Check sheet for the modelled part. Datum: model origin and axes. Units: mm. A direction names the side the tool comes from. Round coordinates to 2 decimals unless told otherwise and drop trailing zeros. Write each loop counter-clockwise with the first axis right and the second up, starting at its lowest first coordinate (ties: lowest second). Pieces come first, ordered by that corner, then holes.
Item 1: Go/stop test with flat-tipped pins: pin 1 Ø1.5 at (y, z) = (5.5, 2.5) entering from +X; pin 2 Ø12.5 at (x, y) = (10.5, -2) entering from -Z; pin 3 Ø2 at (x, z) = (11.5, 2) entering from -Y; pin 4 Ø2.5 at (x, z) = (5.5, 3) entering from +Y. Record where each tip stops, or that it passes through.
Item 2: Cross-section at A-A on x = 0. Enter the section's corners in (y, z), plus the area to 3 significant figures.
Item 3: Cross-section at B-B on z = 8.25. Enter the section's corners in (x, y), plus the area to 3 significant figures.
Item 4: Release check for a two-part mould opening along X. For faces 1 (the flat face through (6, 4.031, 3)), 2 (the cylindrical face through (44.2, -15.6, 6.5)), 3 (the cylindrical face through (20.017, 0.08, 2.958)) record: +X half, -X half, draft (parallel to the pull), parting line (faces both ways), or undercut.
Item 5: Tool access check on faces 4 (the flat face through (43.318, 10.972, 7.521)), 5 (the flat face through (25.915, -11.665, 6.465)), 6 (the cylindrical face through (1.27, -0.97, 7.48)), 7 (the cylindrical face through (0.08, -5.57, 2.96)). Record the directions out of +Z, -Z, +X, -X, +Y, -Y that give a thin tool (end or side, any length) a straight path to the whole face; none if there is none.
Item 6: Cross-section at C-C on y = 0. Enter the section's corners in (x, z).
Item 7: Material ranges on line 1 (Y direction, x = 39.5, z = 7.5); line 2 (Z direction, x = -3.5, y = 1); line 3 (Z direction, x = 17, y = 7), recorded low to high.
from build123d import *

# Parameters (mm, degrees)
BOSS_EXTRUDE1_DEPTH     = 9
BOSS_EXTRUDE2_START     = -5
BOSS_EXTRUDE2_OUTLINE_R = 2.142705637
BOSS_EXTRUDE2_DEPTH     = 5
CUT_EXTRUDE1_DEPTH      = 6
SKETCH9_R               = 1.6
CUT_EXTRUDE2_DEPTH      = 6
CUT_EXTRUDE3_DEPTH      = 3
FILLET1_R               = 1


# Read off the part's stored shape, not the designer's step: Boss-Extrude2
with BuildPart() as part:
    # Sketch2 → Boss-Extrude1 (new body)
    with BuildSketch(Plane.XY):
        with BuildLine():
            Line((13.923486695, -6.250000093), (23.935808117, -6))
            ThreePointArc((23.935808117, -6), (29.935808117, 0), (23.935808117, 6))
            Line((23.935808117, 6), (13.923486695, 6.250000093))
            ThreePointArc((13.923486695, 6.250000093), (9.518581948, 6.542551177), (5.493579732, 8.355871093))
            ThreePointArc((5.493579732, 8.355871093), (-10, 0), (5.493579732, -8.355871093))
            ThreePointArc((5.493579732, -8.355871093), (9.518581948, -6.542551177), (13.923486695, -6.250000093))
        make_face()
    extrude(amount=BOSS_EXTRUDE1_DEPTH)

    # Boss-Extrude2 outline → Boss-Extrude2 (add)
    with BuildSketch(Plane.XY.offset(9).offset(BOSS_EXTRUDE2_START)):
        with BuildLine():
            Line((23.935808117, -6), (13.923486695, -6.250000093))
            Line((13.923486695, -6.250000093), (38.246061815, -17.232807658))
            ThreePointArc((38.246061815, -17.232807658), (44.232088174, -15.557320072), (43.673854661, -9.366347162))
            Line((43.673854661, -9.366347162), (34.3075075, 0))
            Line((34.3075075, 0), (43.673854661, 9.366347162))
            ThreePointArc((43.673854661, 9.366347162), (44.232088174, 15.557320072), (38.246061815, 17.232807658))
            Line((38.246061815, 17.232807658), (13.923486695, 6.250000093))
            Line((13.923486695, 6.250000093), (23.935808117, 6))
            ThreePointArc((23.935808117, 6), (29.935808117, 0), (23.935808117, -6))
        make_face()
        with Locations((40.232073655, -12.797343053)):
            Circle(BOSS_EXTRUDE2_OUTLINE_R, mode=Mode.SUBTRACT)
        with Locations((40.232073655, 12.797343053)):
            Circle(BOSS_EXTRUDE2_OUTLINE_R, mode=Mode.SUBTRACT)
    extrude(amount=BOSS_EXTRUDE2_DEPTH)

    # Sketch7 → Cut-Extrude1 (cut)
    with BuildSketch(Plane(origin=(0, 0, 0), x_dir=(-1, 0, 0), z_dir=(0, 0, -1))):
        with BuildLine():
            ThreePointArc((9.235665873, -3.834380769), (9.999935569, 0.035897224), (9.207899302, 3.900588474))
            Line((9.207899302, 3.900588474), (8.401819085, 4.030860156))
            Line((8.401819085, 4.030860156), (3.901819085, 4.030860156))
            ThreePointArc((3.901819085, 4.030860156), (-0.017364504, 5.630860156), (-3.936548092, 4.030860156))
            Line((-3.936548092, 4.030860156), (-8.436548092, 4.030860156))
            Line((-8.436548092, 4.030860156), (-17.916217693, 2.498838303))
            ThreePointArc((-17.916217693, 2.498838303), (-20.017364504, 0.030860156), (-17.916217693, -2.43711799))
            Line((-17.916217693, -2.43711799), (-8.436548092, -3.969139844))
            Line((-8.436548092, -3.969139844), (-3.936548092, -3.969139844))
            ThreePointArc((-3.936548092, -3.969139844), (-0.017364504, -5.569139844), (3.901819085, -3.969139844))
            Line((3.901819085, -3.969139844), (8.401819085, -3.969139844))
            Line((8.401819085, -3.969139844), (9.235665873, -3.834380769))
        make_face()
    extrude(amount=-CUT_EXTRUDE1_DEPTH, mode=Mode.SUBTRACT)

    # Sketch9 → Cut-Extrude2 (cut)
    with BuildSketch(Plane(origin=(0, 0, 6), x_dir=(-1, 0, 0), z_dir=(0, 0, -1))):
        Circle(SKETCH9_R)
    extrude(amount=-CUT_EXTRUDE2_DEPTH, mode=Mode.SUBTRACT)

    # Sketch10 → Cut-Extrude3 (cut)
    with BuildSketch(Plane.XY.offset(9)):
        Polygon((38.132073655, 9.197343053), (42.332073655, 9.197343053), (44.332073655, 12.797343053), (42.332073655, 16.397343053), (38.132073655, 16.397343053), (36.132073655, 12.797343053), align=None)
        Polygon((38.132073655, -9.197343053), (36.132073655, -12.797343053), (38.132073655, -16.397343053), (42.332073655, -16.397343053), (44.332073655, -12.797343053), (42.332073655, -9.197343053), align=None)
    extrude(amount=-CUT_EXTRUDE3_DEPTH, mode=Mode.SUBTRACT)

    # Fillet1
    fillet1_edges = [part.edges().sort_by_distance(p)[0] for p in [
        (34.3075075, 0, 6.5),
    ]]
    fillet(fillet1_edges, radius=FILLET1_R)


solid = part.part
Response values:
1. pin 1: stops at x = 27.6
1. pin 2: stops at z = 0
1. pin 3: stops at y = -6.34
1. pin 4: stops at y = 9.05
2. outline: (-10, 0) - (-5.57, 0) - (-5.57, 6) - (-1.6, 6) - (-1.6, 9) - (-10, 9) - close; (1.6, 6) - (5.63, 6) - (5.63, 0) - (10, 0) - (10, 9) - (1.6, 9) - close
2. area: 103 mm2
3. outline: (5.49, -8.36) arc R12.43 cw to (13.92, -6.25) - (38.25, -17.23) arc R4.86 ccw to (43.67, -9.37) - (35.01, -0.71) arc R1 cw to (35.01, 0.71) - (43.67, 9.37) arc R4.86 ccw to (38.25, 17.23) - (13.92, 6.25) arc R12.43 cw to (5.49, 8.36) arc R10 ccw (long way) to start; hole circle Ø3.2 at (0, 0); hole (36.13, -12.8) - (38.13, -16.4) - (42.33, -16.4) - (44.33, -12.8) - (42.33, -9.2) - (38.13, -9.2) - close; hole (36.13, 12.8) - (38.13, 9.2) - (42.33, 9.2) - (44.33, 12.8) - (42.33, 16.4) - (38.13, 16.4) - close
3. area: 963 mm2
4. face 1: undercut
4. face 2: parting line
4. face 3: -X half
5. face 4: +Z
5. face 5: +Z, -Z, -Y
5. face 6: +Z, -Z
5. face 7: -Z
6. outline: (-10, 6) - (-1.6, 6) - (-1.6, 9) - (-10, 9) - close; (1.6, 6) - (20.02, 6) - (20.02, 0) - (29.94, 0) - (29.94, 4) - (34.72, 4) - (34.72, 9) - (1.6, 9) - close
7. line 1: y = -17.6 to -16.4, -9.2 to -5.19, 5.19 to 9.2, 16.4 to 17.6
7. line 2: z = 6 to 9
7. line 3: z = 4 to 9
